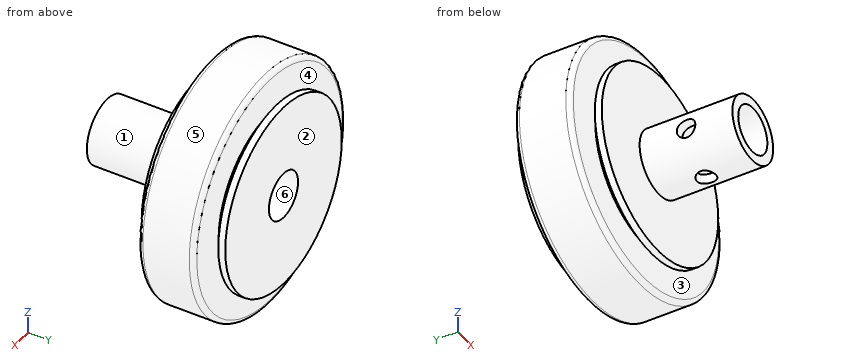
from build123d import *

# Parameters (mm, degrees)
SKETCH_1_R          = 26
EXTRUDE_1_DEPTH     = 12
SKETCH_2_R          = 17.5
EXTRUDE_2_DEPTH     = 1.5
EXTRUDE_START       = 1.5
SKETCH_3_R          = 17.5
EXTRUDE_3_DEPTH     = 1.5
SKETCH_4_R          = 20
EXTRUDE_4_DEPTH     = 1.5
SKETCH_5_R          = 20
EXTRUDE_5_DEPTH     = 1.5
SKETCH_6_R          = 5
CUT_EXTRUDE_1_DEPTH = 41.938978981
EXTRUDE_START_2     = 20
SKETCH_7_R          = 7
SKETCH_7_R_2        = 5
EXTRUDE_6_DEPTH     = 20
SKETCH_8_R          = 2
CUT_EXTRUDE_2_DEPTH = 44.370496884
SKETCH_9_R          = 2
CUT_EXTRUDE_3_DEPTH = 44.370496937
FILLET_1_R          = 1
FILLET_2_R          = 1


with BuildPart() as part:
    # 草图1 → 凸台-拉伸1 (new body)
    with BuildSketch(Plane(origin=(0, 0, 0), x_dir=(1, 0, 0), z_dir=(0, 1, 0))):
        with Locations(Location((0, 0, 0), (0, 0, 270))):
            Circle(SKETCH_1_R)
    extrude(amount=EXTRUDE_1_DEPTH)

    # 草图2 → 凸台-拉伸2 (add)
    with BuildSketch(Plane(origin=(0, 12, 0), x_dir=(1, 0, 0), z_dir=(0, 1, 0))):
        with Locations(Location((0, 0, 0), (0, 0, 270))):
            Circle(SKETCH_2_R)
    extrude(amount=EXTRUDE_2_DEPTH)

    # 草图3 → 凸台-拉伸3 (add)
    with BuildSketch(Plane.XZ.offset(EXTRUDE_START)):
        with Locations(Location((0, 0, 0), (0, 0, 90))):
            Circle(SKETCH_3_R)
    extrude(amount=-EXTRUDE_3_DEPTH)

    # 草图4 → 凸台-拉伸4 (add)
    with BuildSketch(Plane(origin=(0, 13.5, 0), x_dir=(1, 0, 0), z_dir=(0, 1, 0))):
        with Locations(Location((0, 0, 0), (0, 0, 270))):
            Circle(SKETCH_4_R)
    extrude(amount=EXTRUDE_4_DEPTH)

    # 草图5 → 凸台-拉伸5 (add)
    with BuildSketch(Plane.XZ.offset(1.5).offset(EXTRUDE_START)):
        with Locations(Location((0, 0, 0), (0, 0, 90))):
            Circle(SKETCH_5_R)
    extrude(amount=-EXTRUDE_5_DEPTH)

    # 草图6 → 切除-拉伸1 (cut, through all)
    with BuildSketch(Plane.XZ.offset(3)):
        with Locations(Location((0, 0, 0), (0, 0, 270))):
            Circle(SKETCH_6_R)
    extrude(amount=-CUT_EXTRUDE_1_DEPTH, mode=Mode.SUBTRACT)

    # 草图7 → 凸台-拉伸6 (add)
    with BuildSketch(Plane.XZ.offset(3).offset(EXTRUDE_START_2)):
        with Locations(Location((0, 0, 0), (0, 0, 270))):
            Circle(SKETCH_7_R)
        with Locations(Location((0, 0, 0), (0, 0, 270))):
            Circle(SKETCH_7_R_2, mode=Mode.SUBTRACT)
    extrude(amount=-EXTRUDE_6_DEPTH)

    # 草图8 → 切除-拉伸2 (cut, through all)
    with BuildSketch(Plane(origin=(0, 0, 0), x_dir=(0, 0, -1), z_dir=(1, 0, 0))):
        with Locations((0, -13)):
            Circle(SKETCH_8_R)
    extrude(amount=-CUT_EXTRUDE_2_DEPTH, mode=Mode.SUBTRACT)

    # 草图9 → 切除-拉伸3 (cut, through all)
    with BuildSketch(Plane.XY):
        with Locations(Location((0, -13, 0), (0, 0, 270.00000003))):
            Circle(SKETCH_9_R)
    extrude(amount=-CUT_EXTRUDE_3_DEPTH, mode=Mode.SUBTRACT)

    # 圆角1
    fillet_1_edges = [part.edges().sort_by_distance(p)[0] for p in [
        (0, 12, -26),
    ]]
    fillet(fillet_1_edges, radius=FILLET_1_R)

    # 圆角2
    fillet_2_edges = [part.edges().sort_by_distance(p)[0] for p in [
        (0, 0, -26),
    ]]
    fillet(fillet_2_edges, radius=FILLET_2_R)


solid = part.part
The model under review builds one solid part; all positions refer to its coordinate system, in mm. Face numbers are marked on the shaded views. A direction names the side the tool comes from. Coordinates: 2 decimals unless noted, no trailing zeros. Loops run counter-clockwise (first coordinate to the right, second up) from the corner with the lowest first, then second, coordinate; pieces in that order, holes last. Notation, with made-up numbers: M 9.5,15 L 21.5,15 A15 cw 21.5,42 Z; hole C 50.5,38 d8. An arc over 180 degrees is marked long. Put each result on its own line as item: value. Start each with the question number.
Q1. The part is to be moulded in two halves that separate along Z. For the marked faces 4, 5 and 6, say which applies: +Z half, -Z half, draft (parallel to the pull), parting line (faces both ways), or undercut.
Q2. Add section A-A (y = -14). Write out the cut boundary in (x, z).
Q3. Clearance check with flat-ended pins moving along their axes: pin 1 (10 mm diameter, centred on y = -7.5, z = 7.5, fed in from -X); pin 2 (3 mm diameter, centred on x = 0, y = -13, fed in from -Z); pin 3 (10 mm diameter, centred on x = -9, z = -2.5, fed in from -Y); pin 4 (12 mm diameter, centred on y = 9, z = -1, fed in from +X). State where each tip first meets the part, or that it passes through.
Q4. For the marked faces 1, 2 and 3, list the 3-axis set-ups (+Z, -Z, +X, -X, +Y, -Y) from which the entire face can be reached by the end or side of a thin tool; tool diameter is ignored.
Q5. Add section B-B (z = 0). Count the separate pieces of the cut face and the enclosed holes in it, and give its area (3 significant figures).
Q6. Add section D-D (y = -5). Write out the cut boundary in (x, z).
Q7. Wall thickness on line 1 (Y direction, x = 16, z = -9.5); line 2 (X direction, y = -4.5, z = 0); line 3 (Z direction, x = 3, y = 6): over which ranges is each line inside the solid? List them lowest first.
Answers:
1. face 4: draft
1. face 5: parting line
1. face 6: undercut
2. outline: M -6.78,-1.73 A7 ccw -1.73,-6.78 L -1.73,-4.69 A5 cw -4.69,-1.73 Z; M -6.78,1.73 L -4.69,1.73 A5 cw long 1.73,-4.69 L 1.73,-6.78 A7 ccw long Z
3. pin 1: stops at x = -19.28
3. pin 2: stops at z = 4.77
3. pin 3: stops at y = -23
3. pin 4: stops at x = 26
4. face 1: -Y
4. face 2: +Z, -Z, +X, -X, +Y
4. face 3: none
5. separate pieces: 3
5. enclosed holes: 0
5. area: 740 mm^2
6. outline: C 0,0 d14; hole C 0,0 d10
7. line 1: y = -3 to -1.5, 0 to 12, 13.5 to 15
7. line 2: x = -7 to -5, 5 to 7
7. line 3: z = -25.83 to -4, 4 to 25.83
